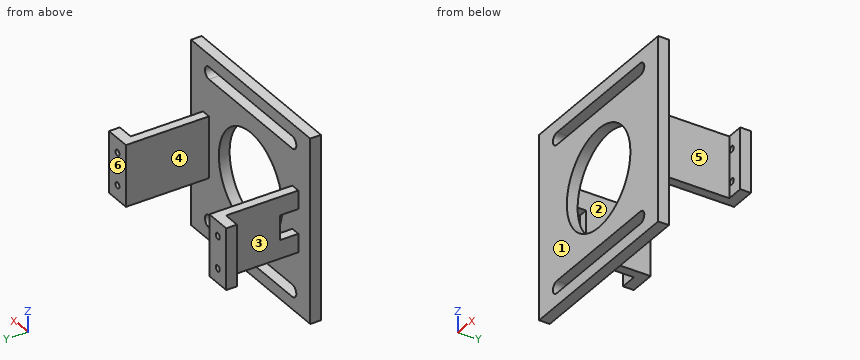
```python
from build123d import *

# Parameters (mm, degrees)
CROQUIS1_W              = 60
CROQUIS1_H              = 60
SALIENTE_EXTRUIR1_DEPTH = 3.5
CROQUIS2_W              = 3
CROQUIS2_H              = 20
SALIENTE_EXTRUIR4_DEPTH = 27
CROQUIS7_R              = 16
CORTAR_EXTRUIR2_DEPTH   = 5
CORTAR_EXTRUIR3_DEPTH   = 5
CROQUIS9_W              = 20
CROQUIS9_H              = 3.5
SALIENTE_EXTRUIR5_DEPTH = 5.5
CROQUIS10_W             = 20
CROQUIS10_H             = 3.5
SALIENTE_EXTRUIR6_DEPTH = 5.5
CROQUIS11_R             = 1
CORTAR_EXTRUIR4_DEPTH   = 5.5
CROQUIS13_R             = 1
CORTAR_EXTRUIR5_DEPTH   = 5.5
CROQUIS14_W             = 8
CROQUIS14_H             = 6
CORTAR_EXTRUIR6_DEPTH   = 10


with BuildPart() as part:
    # Croquis1 → Saliente-Extruir1 (new body)
    with BuildSketch(Plane(origin=(0, 0, 0), x_dir=(1, 0, 0), z_dir=(0, 1, 0))):
        with Locations((-19.589863428, 8.689761392)):
            Rectangle(CROQUIS1_W, CROQUIS1_H)
    extrude(amount=SALIENTE_EXTRUIR1_DEPTH)

    # Croquis2 → Saliente-Extruir4 (add)
    with BuildSketch(Plane(origin=(0, 3.5, 0), x_dir=(1, 0, 0), z_dir=(0, 1, 0))):
        with Locations((2.910136572, 8.689761392)):
            Rectangle(CROQUIS2_W, CROQUIS2_H)
        with Locations((-42.089863428, 8.689761392)):
            Rectangle(CROQUIS2_W, CROQUIS2_H)
    extrude(amount=SALIENTE_EXTRUIR4_DEPTH)

    # Croquis7 → Cortar-Extruir2 (cut)
    with BuildSketch(Plane(origin=(0, 3.5, 0), x_dir=(1, 0, 0), z_dir=(0, 1, 0))):
        with Locations(Location((-19.589863428, 8.689761392, 0), (0, 0, 270))):
            Circle(CROQUIS7_R)
    extrude(amount=-CORTAR_EXTRUIR2_DEPTH, mode=Mode.SUBTRACT)

    # Croquis8 → Cortar-Extruir3 (cut)
    with BuildSketch(Plane(origin=(0, 3.5, 0), x_dir=(1, 0, 0), z_dir=(0, 1, 0))):
        with BuildLine():
            Line((1.410136572, -17.310238608), (-40.589863428, -17.310238608))
            ThreePointArc((-40.589863428, -17.310238608), (-42.589863428, -15.310238608), (-40.589863428, -13.310238608))
            Line((-40.589863428, -13.310238608), (1.410136572, -13.310238608))
            ThreePointArc((1.410136572, -13.310238608), (3.410136572, -15.310238608), (1.410136572, -17.310238608))
        make_face()
        with BuildLine():
            Line((1.410136572, 30.689761392), (-40.589863428, 30.689761392))
            ThreePointArc((-40.589863428, 30.689761392), (-42.589863428, 32.689761392), (-40.589863428, 34.689761392))
            Line((-40.589863428, 34.689761392), (1.410136572, 34.689761392))
            ThreePointArc((1.410136572, 34.689761392), (3.410136572, 32.689761392), (1.410136572, 30.689761392))
        make_face()
    extrude(amount=-CORTAR_EXTRUIR3_DEPTH, mode=Mode.SUBTRACT)

    # Croquis9 → Saliente-Extruir5 (add)
    with BuildSketch(Plane(origin=(4.410136572, 0, 0), x_dir=(0, 0, -1), z_dir=(1, 0, 0))):
        with Locations((8.689761392, 28.75)):
            Rectangle(CROQUIS9_W, CROQUIS9_H)
    extrude(amount=SALIENTE_EXTRUIR5_DEPTH)

    # Croquis10 → Saliente-Extruir6 (add)
    with BuildSketch(Plane.ZY.offset(43.589863428)):
        with Locations((-8.689761392, 28.75)):
            Rectangle(CROQUIS10_W, CROQUIS10_H)
    extrude(amount=SALIENTE_EXTRUIR6_DEPTH)

    # Croquis11 → Cortar-Extruir4 (cut)
    with BuildSketch(Plane(origin=(0, 30.5, 0), x_dir=(1, 0, 0), z_dir=(0, 1, 0))):
        with Locations(Location((-44.839863428, 3.439761392, 0), (0, 0, 270))):
            Circle(CROQUIS11_R)
        with Locations(Location((-44.839863428, 13.939761392, 0), (0, 0, 270))):
            Circle(CROQUIS11_R)
    extrude(amount=-CORTAR_EXTRUIR4_DEPTH, mode=Mode.SUBTRACT)

    # Croquis13 → Cortar-Extruir5 (cut)
    with BuildSketch(Plane(origin=(0, 30.5, 0), x_dir=(1, 0, 0), z_dir=(0, 1, 0))):
        with Locations(Location((5.660136572, 3.439761392, 0), (0, 0, 270))):
            Circle(CROQUIS13_R)
        with Locations(Location((5.660136572, 13.939761392, 0), (0, 0, 270))):
            Circle(CROQUIS13_R)
    extrude(amount=-CORTAR_EXTRUIR5_DEPTH, mode=Mode.SUBTRACT)

    # Croquis14 → Cortar-Extruir6 (cut)
    with BuildSketch(Plane.ZY.offset(43.589863428)):
        with Locations((-8.689761392, 6.5)):
            Rectangle(CROQUIS14_W, CROQUIS14_H)
    extrude(amount=-CORTAR_EXTRUIR6_DEPTH, mode=Mode.SUBTRACT)


solid = part.part
```
Geometry: final body of the model. Coordinates: model frame, mm. Face numbers are marked on the shaded views. A direction names the side the tool comes from. Round coordinates to 2 decimals unless told otherwise and drop trailing zeros. Order: outer loops, then holes, each group sorted by start corner. A loop starts at its lowest first (then second) coordinate and runs counter-clockwise, first axis right, second up. Notation, with made-up numbers: (76, 80) - (100, 80) arc R22 ccw to (100, 88) - close; hole circle Ø11 at (3.25, 82.5). An arc over 180 degrees is marked (long way). Use CSV: the item, a comma, the result in double quotes. Start each with the question number.
Q1. Section query A-A (x = -2). Return loops of the section in (y, z).
Q2. Mould query, pull axis Y, two halves, no side actions, for the marked faces 4, 5 and 6. Classes: +Y half, -Y half, draft (parallel to the pull), parting line (faces both ways), or undercut.
Q3. Material intervals for line 1 along X through (y, z) = (12, -14); line 2 along Y through (x, z) = (-46, 17); line 3 along X through (y, z) = (27.5, -15), sorted ascending. Write a range as from..to.
Q4. Access query for the marked faces 1, 2 and 3. Directions: +Z, -Z, +X, -X, +Y, -Y. A direction counts if a zero-diameter tool reaches every point of the face in a straight line with its end or side. Return the directions, or none.
Q5. Section query B-B (y = 25.5). Return loops of the section in (x, z).
Q6. Section query D-D (x = -16). Return loops of the section in (y, z), and give its area (3 significant figures).
Q7. Section query C-C (z = -23). Return loops of the section in (x, y), and give its area (3 significant figures).
Q8. First-contact query: pin 1 (4 mm diameter, centred on x = -45.5, y = 13.5, fed in from +Z); pin 2 (1 mm diameter, centred on x = -20, z = -27.5, fed in from +Y); pin 3 (10 mm diameter, centred on y = 17, z = -5.5, fed in from +X). Flat tips, straight axial feed; report the tip coordinate or a pass-through.
Result set:
1,outline,"(0, -38.69) - (3.5, -38.69) - (3.5, -34.69) - (0, -34.69) - close; (0, -30.69) - (3.5, -30.69) - (3.5, 13.31) - (0, 13.31) - close; (0, 17.31) - (3.5, 17.31) - (3.5, 21.31) - (0, 21.31) - close"
2,face 4,"draft"
2,face 5,"undercut"
2,face 6,"+Y half"
3,line 1,"x = -43.59..-40.59, 1.41..4.41"
3,line 2,"y = 0..3.5"
3,line 3,"x = -49.09..-40.59, 1.41..9.91"
4,face 1,"+Z, -Z, +X, -X, -Y"
4,face 2,"+Z, -Z, +Y"
4,face 3,"+Z, -Z, -X"
5,outline,"(-43.59, -18.69) - (-40.59, -18.69) - (-40.59, 1.31) - (-43.59, 1.31) - close; (1.41, -18.69) - (4.41, -18.69) - (4.41, 1.31) - (1.41, 1.31) - close"
6,outline,"(0, -38.69) - (3.5, -38.69) - (3.5, -34.69) - (0, -34.69) - close; (0, -30.69) - (3.5, -30.69) - (3.5, -24.28) - (0, -24.28) - close; (0, 6.9) - (3.5, 6.9) - (3.5, 13.31) - (0, 13.31) - close; (0, 17.31) - (3.5, 17.31) - (3.5, 21.31) - (0, 21.31) - close"
6,area,"72.9 mm2"
7,outline,"(-49.59, 0) - (-26.75, 0) - (-26.75, 3.5) - (-49.59, 3.5) - close; (-12.43, 0) - (10.41, 0) - (10.41, 3.5) - (-12.43, 3.5) - close"
7,area,"160 mm2"
8,pin 1,"stops at z = 1.31"
8,pin 2,"stops at y = 3.5"
8,pin 3,"stops at x = 4.41"
